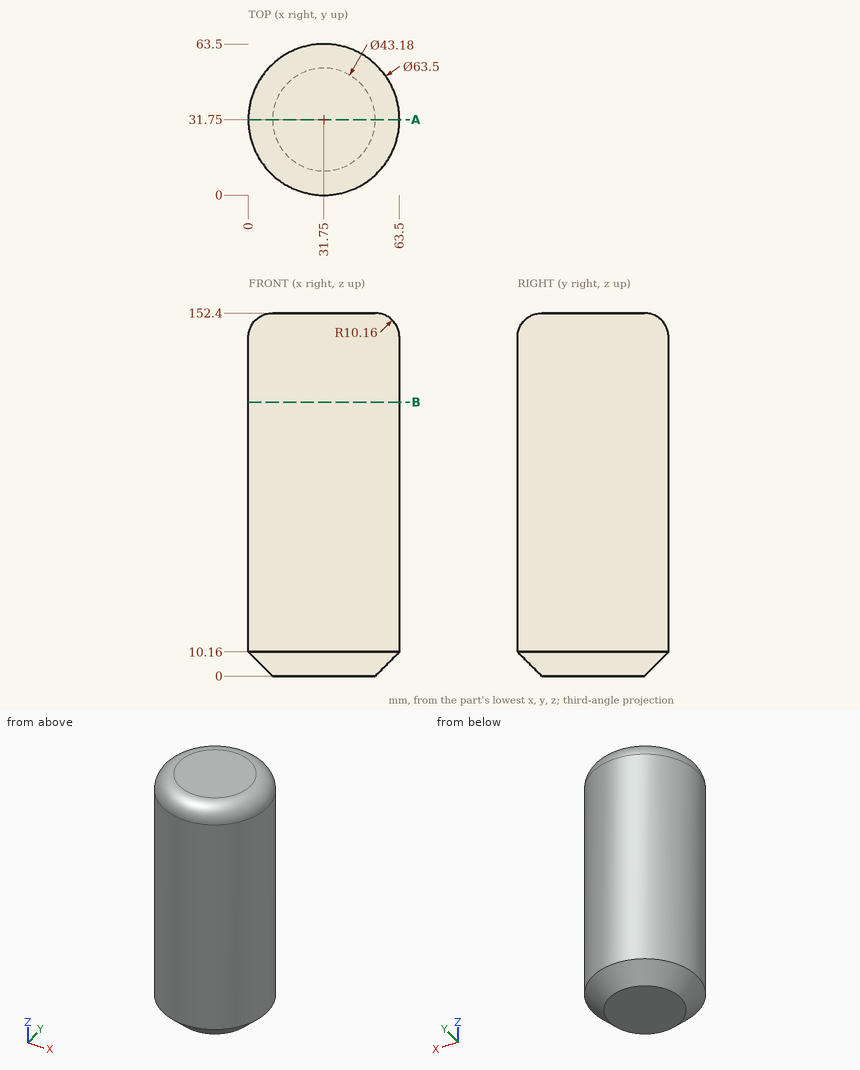
For this review, use the dimensioned drawing (mm, ordinates from the lowest corner) and the shaded views. Coordinates: 2 decimals unless noted, no trailing zeros. Loops run counter-clockwise (first coordinate to the right, second up) from the corner with the lowest first, then second, coordinate; pieces in that order, holes last. Notation, with made-up numbers: (56, -15.75) -> (90, -15.75) arc R36 cw to (90, 20.25) -> close; hole circle Ø8 at (28, -2.5). An arc over 180 degrees is marked (long way). Use a Markdown table: item, result. Add a question column.
Item 1: Clearance check with flat-ended pins moving along their axes: P1, Ø12, axis at x = 18.5, z = 15.5, coming from the +Y side; P2, Ø10, axis at y = 47.5, z = 28, coming from the -X side; P3, Ø6, axis at x = 6.5, z = 68.5, coming from the -Y side. State where each tip first meets the part, or that it passes through.
Item 2: We need section B-B, the plane z = 115. Write out the cut boundary in (x, y), and give its area (3 significant figures).
Item 3: We need section A-A, the plane y = 31.75. Write out the cut boundary in (x, z).
Item 4: Wall thickness on L1, parallel to Y at x = 32.5, z = 83.5; L2, parallel to Y at x = 55, z = 20; L3, parallel to X at y = 41, z = 97: over which ranges is each line inside the solid? List them lowest first. Write a range as from..to.
Numbers:
| question | item | result |
|---|---|---|
| 1 | P1 | stops at y = 62.66 |
| 1 | P2 | stops at x = 1.88 |
| 1 | P3 | stops at y = 9.1 |
| 2 | outline | circle Ø63.5 at (31.75, 31.75) |
| 2 | area | 3,170 mm^2 |
| 3 | outline | (0, 10.16) -> (10.16, 0) -> (53.34, 0) -> (63.5, 10.16) -> (63.5, 142.24) arc R10.16 ccw to (53.34, 152.4) -> (10.16, 152.4) arc R10.16 ccw to (0, 142.24) -> close |
| 4 | L1 | y = 0.01..63.49 |
| 4 | L2 | y = 10.13..53.37 |
| 4 | L3 | x = 1.38..62.12 |
